Source: CAD feature listing. Evaluate the final solid. Frame: model axes, mm. Face numbers are marked on the shaded views. Coordinates: 2 decimals unless noted, no trailing zeros. Order: outer loops, then holes, each group sorted by start corner. A loop starts at its lowest first (then second) coordinate and runs counter-clockwise, first axis right, second up.
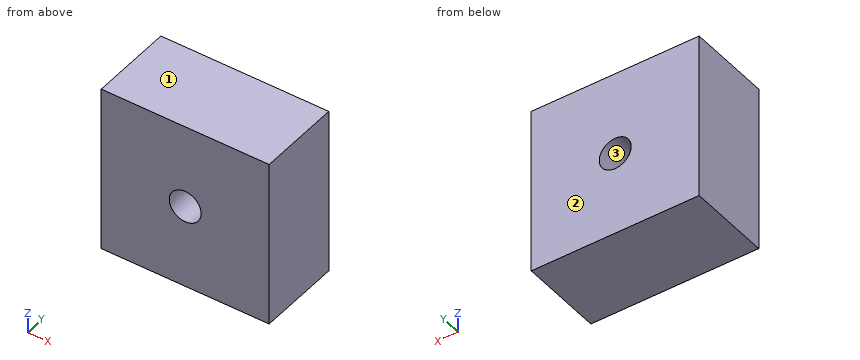
Autodesk Inventor part; units mm, degrees
ref_plane "YZ Plane" through (0, 0, 0) normal (1, 0, 0) x (0, 1, 0)
ref_plane "XZ Plane" through (0, 0, 0) normal (0, 1, 0) x (-1, 0, 0)
ref_plane "XY Plane" through (0, 0, 0) normal (0, 0, 1) x (1, 0, 0)
sketch "Sketch1" plane through (0, 0, 0) normal (0, 1, 0) x (-1, 0, 0)
  line L0 (0, 0) -> (20, 0)
  line L1 (20, 0) -> (20, 20)
  line L2 (20, 20) -> (0, 20)
  line L3 (0, 20) -> (0, 0)
  dimension "d0" = 20
  dimension "d1" = 20
extrude "Extrusion1" add sketch "Sketch1" along normal blind 10
sketch "Sketch2" plane through (0, 10, 0) normal (0, 1, 0) x (1, 0, 0)
  line L0 (0, 0) -> (-20, 0) construction
  line L1 (-10, 0) -> (-10, -20) construction
  line L2 (-20, -20) -> (0, -20) construction
  line L3 (-20, 0) -> (-20, -20) construction
  line L4 (-20, -10) -> (0, -10) construction
  line L5 (0, -20) -> (0, 0) construction
  circle A0 centre (-10, -10) radius 1.9
  dimension "d4" = 3.8
extrude "Extrusion3" cut sketch "Sketch2" against normal blind 20
properties part number "_3DPrint"
Q1. Section query A-A on z = 10. Output: boundary loops of the cut face in (x, y).
Solutions:
outline: (-20, 0) - (-11.9, 0) - (-11.9, 10) - (-20, 10) - close; (-8.1, 0) - (0, 0) - (0, 10) - (-8.1, 10) - close
Q2. Section query C-C on y = 4.25. Output: boundary loops of the cut face in (x, z).
Solutions:
outline: (-20, 0) - (0, 0) - (0, 20) - (-20, 20) - close; hole circle Ø3.8 at (-10, 10)
Q3. Section query B-B on x = -10. Output: boundary loops of the cut face in (y, z), plus the area to 3 significant figures.
Solutions:
outline: (0, 0) - (10, 0) - (10, 8.1) - (0, 8.1) - close; (0, 11.9) - (10, 11.9) - (10, 20) - (0, 20) - close
area: 162 mm2
Q4. Pull-direction query (Z, two-part tool) for the marked faces 1, 2 and 3; classes: pulls with the +Z half, pulls with the -Z half, needs draft (parallel to the pull), parting line crosses it, or undercut.
Solutions:
face 1: pulls with the +Z half
face 2: needs draft
face 3: undercut
Q5. Material intervals for line 1 along X through (y, z) = (4.5, 10); line 2 along Z through (x, y) = (-10, 2.5); line 3 along Z through (x, y) = (-11.5, 6), sorted ascending.
Solutions:
line 1: x = -20 to -11.9, -8.1 to 0
line 2: z = 0 to 8.1, 11.9 to 20
line 3: z = 0 to 8.83, 11.17 to 20
